The model under review builds one solid part; all positions refer to its coordinate system, in mm. A direction names the side the tool comes from. Round coordinates to 2 decimals unless told otherwise and drop trailing zeros. Loops run counter-clockwise (first coordinate to the right, second up) from the corner with the lowest first, then second, coordinate; pieces in that order, holes last. Notation, with made-up numbers: (-33, 21) -> (0, 21) arc R20 ccw to (0, 52) -> close; hole circle Ø8 at (61, 37.25). An arc over 180 degrees is marked (long way). Use CSV: the item, a comma, the result in double quotes. Start each with the question number.
```python
from build123d import *

# Parameters (mm, degrees)
ESQUISSE2_R        = 7.5
BOSS_EXTRU_1_DEPTH = 10
BOSS_EXTRU_2_DEPTH = 5
CONG_2_R           = 5
CONG_3_R           = 2
ESQUISSE4_W        = 5
ESQUISSE4_H        = 110
BOSS_EXTRU_3_DEPTH = 10
SYM_TRIE3_START    = 75
SYM_TRIE3_DEPTH    = 5
ESQUISSE5_R        = 7.5
BOSS_EXTRU_4_DEPTH = 10
CONG_4_START       = -1.578947368
CONG_4_DEPTH       = 22.578947368
CONG_4_START_2     = 15
CONG_4_2_DEPTH     = 5


with BuildPart() as part:
    # Esquisse2 → Boss.-Extru.1 (new body)
    with BuildSketch(Plane(origin=(0, 0, 0), x_dir=(1, 0, 0), z_dir=(0, 1, 0))):
        with Locations(Location((0, 0, 0), (0, 0, 270))):
            Circle(ESQUISSE2_R)
    extrude(amount=BOSS_EXTRU_1_DEPTH)

    # Esquisse3 → Boss.-Extru.2 (add)
    with BuildSketch(Plane(origin=(0, 10, 0), x_dir=(1, 0, 0), z_dir=(0, 1, 0))):
        with BuildLine():
            Line((15, 0), (15, -15))
            Line((15, -15), (70, -15))
            Line((70, -15), (70, -20))
            Line((70, -20), (10, -20))
            Line((10, -20), (10, -7.5))
            Line((10, -7.5), (0, -7.5))
            ThreePointArc((0, -7.5), (-5.303300859, 5.303300859), (7.5, 0))
            Line((7.5, 0), (15, 0))
        make_face()
    extrude(amount=BOSS_EXTRU_2_DEPTH)

    # Congé2
    cong_2_edges = [part.edges().sort_by_distance(p)[0] for p in [
        (10, 12.5, 20),
        (15, 12.5, 15),
        (15, 12.5, 0),
        (10, 12.5, 7.5),
    ]]
    fillet(cong_2_edges, radius=CONG_2_R)

    # Congé3
    cong_3_edges = [part.edges().sort_by_distance(p)[0] for p in [
        (7.5, 12.5, 0),
    ]]
    fillet(cong_3_edges, radius=CONG_3_R)

    # Esquisse4 → Boss.-Extru.3 (add)
    with BuildSketch(Plane(origin=(70, 0, 0), x_dir=(0, 0, -1), z_dir=(1, 0, 0))):
        with Locations((-17.5, 45)):
            Rectangle(ESQUISSE4_W, ESQUISSE4_H)
    extrude(amount=BOSS_EXTRU_3_DEPTH)

    # Symétrie3: read off the stored shape, not the designer's step
    # Symétrie3 outline → Symétrie3 (add)
    with BuildSketch(Plane(origin=(0, 0, 0), x_dir=(1, 0, 0), z_dir=(0, 1, 0)).offset(SYM_TRIE3_START)):
        with BuildLine():
            ThreePointArc((9.287087811, 0), (8.030526086, 0.44402679), (7.331911429, 1.578947368))
            ThreePointArc((7.331911429, 1.578947368), (-5.834899539, 4.712106468), (0, -7.5))
            Line((0, -7.5), (5, -7.5))
            ThreePointArc((5, -7.5), (8.535533906, -8.964466094), (10, -12.5))
            Line((10, -12.5), (10, -15))
            ThreePointArc((10, -15), (11.464466094, -18.535533906), (15, -20))
            Line((15, -20), (70, -20))
            Line((70, -20), (70, -15))
            Line((70, -15), (20, -15))
            ThreePointArc((20, -15), (16.464466094, -13.535533906), (15, -10))
            Line((15, -10), (15, -5))
            ThreePointArc((15, -5), (13.535533906, -1.464466094), (10, 0))
            Line((10, 0), (9.287087811, 0))
        make_face()
    extrude(amount=SYM_TRIE3_DEPTH)

    # Esquisse5 → Boss.-Extru.4 (add)
    with BuildSketch(Plane(origin=(0, 80, 0), x_dir=(1, 0, 0), z_dir=(0, 1, 0))):
        with Locations(Location((0, 0, 0), (0, 0, 270))):
            Circle(ESQUISSE5_R)
    extrude(amount=BOSS_EXTRU_4_DEPTH)

    # Congé4: read off the stored shape, not the designer's step
    # Congé4 outline → Congé4 (cut)
    with BuildSketch(Plane.XY.offset(CONG_4_START)):
        with BuildLine():
            Line((70, -10), (75, -10))
            ThreePointArc((75, -10), (71.464466094, -8.535533906), (70, -5))
            Line((70, -5), (70, -10))
        make_face()
        with BuildLine():
            Line((80, -10), (80, -5))
            ThreePointArc((80, -5), (78.535533906, -8.535533906), (75, -10))
            Line((75, -10), (80, -10))
        make_face()
        with BuildLine():
            Line((80, 100), (75, 100))
            ThreePointArc((75, 100), (78.535533906, 98.535533906), (80, 95))
            Line((80, 95), (80, 100))
        make_face()
        with BuildLine():
            Line((70, 100), (70, 95))
            ThreePointArc((70, 95), (71.464466094, 98.535533906), (75, 100))
            Line((75, 100), (70, 100))
        make_face()
    extrude(amount=CONG_4_DEPTH, mode=Mode.SUBTRACT)

    # Cong_4 2 outline → Cong_4 2 (add)
    with BuildSketch(Plane.XY.offset(CONG_4_START_2)):
        with BuildLine():
            Line((70, 15), (70, 20))
            ThreePointArc((70, 20), (68.535533906, 16.464466094), (65, 15))
            Line((65, 15), (70, 15))
        make_face()
        with BuildLine():
            ThreePointArc((65, 75), (68.535533906, 73.535533906), (70, 70))
            Line((70, 70), (70, 75))
            Line((70, 75), (65, 75))
        make_face()
        with BuildLine():
            Line((70, 80), (70, 85))
            ThreePointArc((70, 85), (68.535533906, 81.464466094), (65, 80))
            Line((65, 80), (70, 80))
        make_face()
        with BuildLine():
            ThreePointArc((65, 10), (68.535533906, 8.535533906), (70, 5))
            Line((70, 5), (70, 10))
            Line((70, 10), (65, 10))
        make_face()
    extrude(amount=CONG_4_2_DEPTH)


solid = part.part
```
1. For faces 4 (the face through (15, 12, 7)), 5 (the face through (69, 17, 17)), 6 (the face through (70, 0, 18)), 7 (the face through (10, 77, 14)), 8 (the face through (0, 0, 0)), list the 3-axis set-ups (+Z, -Z, +X, -X, +Y, -Y) from which the entire face can be reached by the end or side of a thin tool; tool diameter is ignored.
2. The part is to be moulded in two halves that separate along Y. For faces 1 (the face through (69, 82, 17)), 2 (the face through (15, 15, 12)), 3 (the face through (8.5, 12.54, 8.93)), say which applies: pulls with the +Y half, pulls with the -Y half, needs draft (parallel to the pull), parting line crosses it, or undercut.
3. Take a section at B-B, the plane z = -3.5. Give the boundary of the cut face in (x, y), then the cut area to 3 significant figures.
4. For line 1 along Y through (x, z) = (62, 15.25); line 2 along Y through (x, z) = (0, 3); line 3 along X through (y, z) = (76.5, 13), list the stretches that pass through material, from the lowest coordinate up. Write a range as from..to.
5. Clearance check with flat-ended pins moving along their axes: P1, Ø3, axis at y = 10.5, z = 10, coming from the -X side; P2, Ø6, axis at y = 79, z = 2.5, coming from the -X side; P3, Ø12, axis at x = 2, z = 6.5, coming from the -Y side; P4, Ø1.5, axis at y = 90.5, z = 17, coming from the -X side. State where each tip first meets the part, or that it passes through.
6. Take a section at A-A, the plane x = 58.5. Give the boundary of the cut face in (y, z).
7. Take a section at C-C, the plane z = 16.5. Give the boundary of the cut face in (x, y), then the cut area to 3 significant figures.
8. Take a section at D-D, the plane x = 11.5. Give the boundary of the cut face in (y, z), then the cut area to 3 significant figures.
Results:
1,face 4,"-Z, +X, +Y, -Y"
1,face 5,"+Z, -Z, -X"
1,face 6,"+Z, -Z, -X, -Y"
1,face 7,"+Z, -X, +Y, -Y"
1,face 8,"+Z, -Z, +X, -X, -Y"
2,face 1,"pulls with the +Y half"
2,face 2,"undercut"
2,face 3,"needs draft"
3,outline,"(-6.63, 0) -> (6.63, 0) -> (6.63, 15) -> (-6.63, 15) -> close; (-6.63, 75) -> (6.63, 75) -> (6.63, 90) -> (-6.63, 90) -> close"
3,area,"398 mm²"
4,line 1,"10..15, 75..80"
4,line 2,"0..15, 75..90"
4,line 3,"10..16"
5,P1,"x = 8"
5,P2,"x = -7.5"
5,P3,"y = 0"
5,P4,"x = 70"
6,outline,"(10, 15) -> (15, 15) -> (15, 20) -> (10, 20) -> close; (75, 15) -> (80, 15) -> (80, 20) -> (75, 20) -> close"
7,outline,"(10.23, 10) -> (65, 10) arc R5 cw to (70, 5) -> (70, -5) arc R5 ccw to (80, -5) -> (80, 95) arc R5 ccw to (70, 95) -> (70, 85) arc R5 cw to (65, 80) -> (10.23, 80) -> (10.23, 75) -> (65, 75) arc R5 cw to (70, 70) -> (70, 20) arc R5 cw to (65, 15) -> (10.23, 15) -> close"
7,area,"1,700 mm²"
8,outline,"(10, 0.23) -> (15, 0.23) -> (15, 18.57) -> (10, 18.57) -> close; (75, 0.23) -> (80, 0.23) -> (80, 18.57) -> (75, 18.57) -> close"
8,area,"183 mm²"
